The drawing under review shows one solid part. Ordinate dimensions are in mm from its lowest x, y, z. Round coordinates to 2 decimals unless told otherwise and drop trailing zeros. Order: outer loops, then holes, each group sorted by start corner. A loop starts at its lowest first (then second) coordinate and runs counter-clockwise, first axis right, second up. Notation, with made-up numbers: (4, 81) -> (11, 81) arc R31 ccw to (11, 110) -> close; hole circle Ø7 at (-26.75, 70.5). An arc over 180 degrees is marked (long way). Return JSON: item names as keys, results as strings. Group by question number.
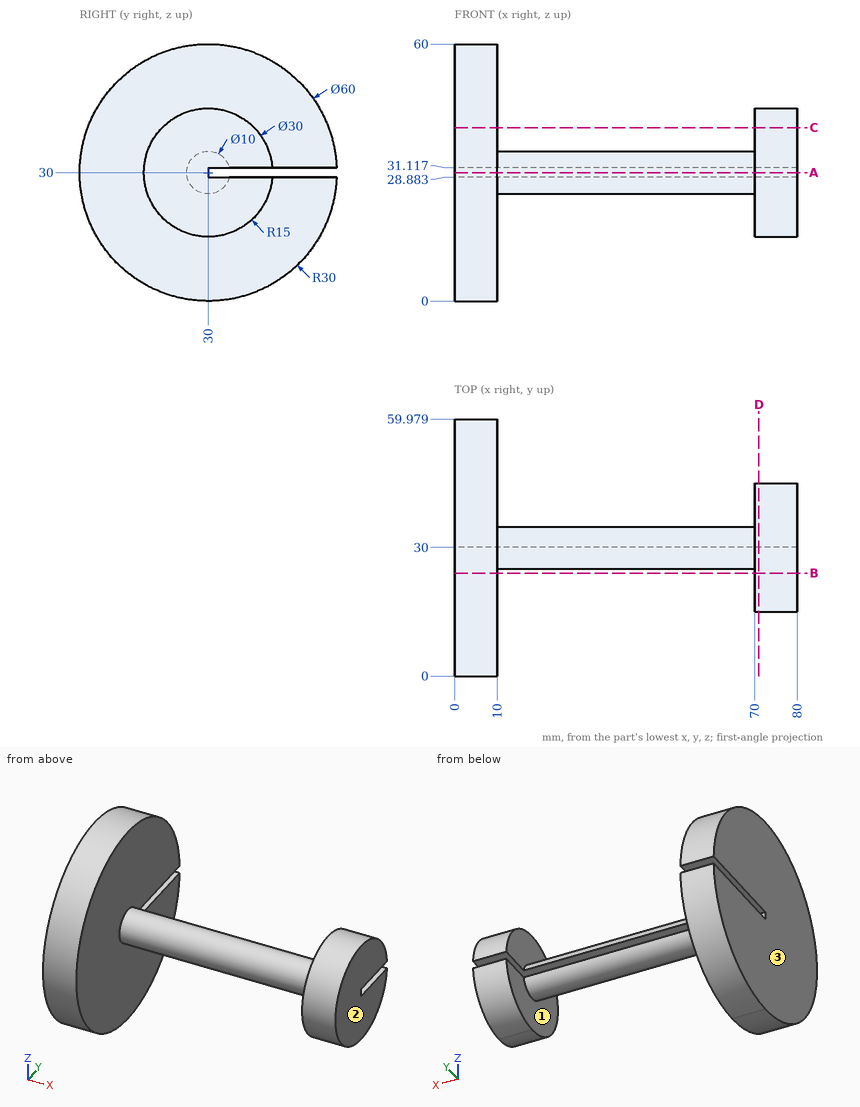
Item 1: Wall thickness on line 1 along X through (y, z) = (41, 21.5); line 2 along X through (y, z) = (48, 31.5); line 3 along Z through (x, y) = (53, 31): over which ranges is each line inside the solid? List them lowest first.
Item 2: Insertion check: pin 1 Ø2 at (x, y) = (36, 26.5) entering from +Z; pin 2 Ø9 at (x, y) = (48, 37.5) entering from -Z; pin 3 Ø12 at (x, y) = (10.5, 9.5) entering from -Z. Each pin has a flat end and moves straight along its axis. Give the tip position at first contact, or say it passes through.
Item 3: Consider section B-B on y = 24. State the section outline as (x, z) points, plus the area to 3 significant figures.
Item 4: Consider section C-C on z = 40.5. State the section outline as (x, y) points, plus the area to 3 significant figures.
Item 5: The part is to be moulded in two halves that separate along X. For the marked faces 1, 2 and 3, say which applies: +X half, -X half, draft (parallel to the pull), parting line (faces both ways), or undercut.
Item 6: Consider section D-D on x = 71. State the section outline as (y, z) points.
Item 7: Consider section A-A on z = 30. State the section outline as (x, y) points.
Values:
{
 "1": {"line 1": "0 to 10, 70 to 80", "line 2": "0 to 10", "line 3": "25.1 to 28.88, 31.12 to 34.9"},
 "2": {"pin 1": "z = 34.33", "pin 2": "z = 26", "pin 3": "z = 3.75"},
 "3": {"outline": "(0, 0.61) -> (10, 0.61) -> (10, 59.39) -> (0, 59.39) -> close; (70, 16.25) -> (80, 16.25) -> (80, 43.75) -> (70, 43.75) -> close", "area": "863 mm^2"},
 "4": {"outline": "(0, 1.9) -> (10, 1.9) -> (10, 58.1) -> (0, 58.1) -> close; (70, 19.29) -> (80, 19.29) -> (80, 40.71) -> (70, 40.71) -> close", "area": "776 mm^2"},
 "5": {"face 1": "undercut", "face 2": "+X half", "face 3": "-X half"},
 "6": {"outline": "(30, 28.88) -> (30, 31.12) -> (44.96, 31.12) arc R15 ccw (long way) to (44.96, 28.88) -> close"},
 "7": {"outline": "(0, 0) -> (10, 0) -> (10, 25) -> (70, 25) -> (70, 15) -> (80, 15) -> (80, 30) -> (0, 30) -> close"}
}
